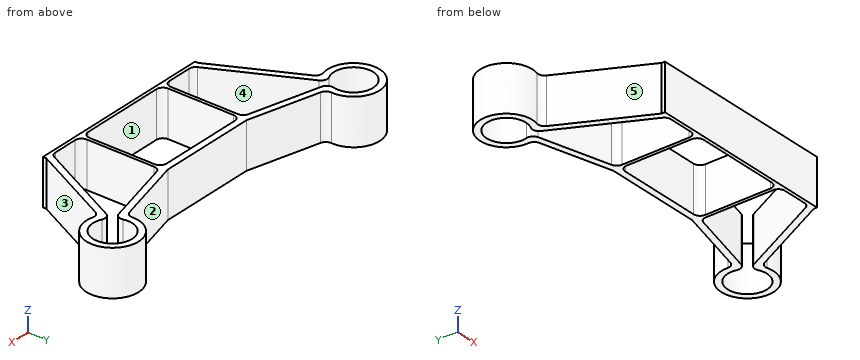
```python
from build123d import *

# Parameters (mm, degrees)
F1_DEPTH = 7
F2_R     = 1
F3_R     = 1


with BuildPart() as f1:
    # F0 (on Top) → F1 (new body)
    with BuildSketch(Plane.XY):
        with BuildLine():
            ThreePointArc((20.490715, 21.30806), (25.314352, 24.866528), (20.822566, 20.897394))
            Line((20.822566, 20.897394), (13.382216, 6))
            Line((13.382216, 6), (14.5, 6))
            Line((14.5, 6), (21.19372, 19.40246))
            ThreePointArc((21.19372, 19.40246), (26.092146, 25.495048), (19.107008, 21.984771))
            Line((19.107008, 21.984771), (7.5, 19))
            Line((7.5, 19), (0, 19))
            Line((0, 19), (0, 18))
            Line((0, 18), (7.5, 18))
            Line((7.5, 18), (7.626518, 18))
            Line((7.626518, 18), (8, 18.096042))
            Line((8, 18.096042), (20.490715, 21.30806))
        make_face()
        Polygon((14.5, 6), (13.382216, 6), (8, 6), (7.5, 6), (0, 6), (0, 5.5), (14.5, 5.5), align=None)
        Polygon((8, 6), (8, 18.096042), (7.626518, 18), (7.5, 18), (7.5, 6), align=None)
    extrude(amount=F1_DEPTH)

    # F2
    f2_edges = [f1.edges().sort_by_distance(p)[0] for p in [
        (21.19372, 19.40246, 3.5),
        (20.822566, 20.897394, 3.5),
        (20.490715, 21.30806, 3.5),
        (19.107008, 21.984771, 3.5),
    ]]
    fillet(f2_edges, radius=F2_R)

    # F3
    f3_edges = [f1.edges().sort_by_distance(p)[0] for p in [
        (8, 18.096042, 3.5),
        (13.382216, 6, 3.5),
        (8, 6, 3.5),
        (7.5, 18, 3.5),
        (7.5, 6, 3.5),
    ]]
    fillet(f3_edges, radius=F3_R)

    # F4: F1 across plane


with BuildPart() as f1_1:
    add(f1.part)
    add(f1.part.mirror(Plane.YZ))


solid = f1_1.part
```
Design review of the part built by this model. Coordinates are the model's own, in mm. Face numbers are marked on the shaded views. A direction names the side the tool comes from. Round coordinates to 2 decimals unless told otherwise and drop trailing zeros. Write each loop counter-clockwise with the first axis right and the second up, starting at its lowest first coordinate (ties: lowest second). Pieces come first, ordered by that corner, then holes. Notation, with made-up numbers: (-8.5, 40) -> (39.5, 40) arc R22 cw to (39.5, 59) -> close; hole circle Ø1 at (33, 85.5). An arc over 180 degrees is marked (long way). Answer in a Markdown table with one row per item.
Q1. To check wall thickness, follow L1, parallel to X at y = 11.5, z = 4.5; L2, parallel to Y at x = 3, z = 0.75; L3, parallel to X at y = 24.25, z = 6. State the ranges of each line that lie inside material, in increasing order. Write a range as [from, to].
The answers:
| item | result |
|---|---|
| L1 | [-17.25, -16.13], [-8, -7.5], [7.5, 8], [16.13, 17.25] |
| L2 | [5.5, 6], [18, 19] |
| L3 | [-26.77, -25.7], [-20.26, -19.19], [19.19, 20.26], [25.7, 26.77] |
Q2. Take a section at B-B, the plane y = 23.25. State the section outline as (x, z) points, then the cut area to 3 significant figures.
The answers:
| item | result |
|---|---|
| outline | (-26.97, 0) -> (-25.97, 0) -> (-25.97, 7) -> (-26.97, 7) -> close; (-19.99, 0) -> (-18.99, 0) -> (-18.99, 7) -> (-19.99, 7) -> close; (18.99, 0) -> (19.99, 0) -> (19.99, 7) -> (18.99, 7) -> close; (25.97, 0) -> (26.97, 0) -> (26.97, 7) -> (25.97, 7) -> close |
| area | 28.1 mm² |
Q3. Take a section at D-D, the plane y = 16.25. State the section outline as (x, z) points, then the cut area to 3 significant figures.
The answers:
| item | result |
|---|---|
| outline | (-19.62, 0) -> (-18.5, 0) -> (-18.5, 7) -> (-19.62, 7) -> close; (-8, 0) -> (-7.5, 0) -> (-7.5, 7) -> (-8, 7) -> close; (7.5, 0) -> (8, 0) -> (8, 7) -> (7.5, 7) -> close; (18.5, 0) -> (19.62, 0) -> (19.62, 7) -> (18.5, 7) -> close |
| area | 22.6 mm² |
Q4. Take a section at A-A, the plane x = 1. State the section outline as (y, z) points, then the cut area to 3 significant figures.
The answers:
| item | result |
|---|---|
| outline | (5.5, 0) -> (6, 0) -> (6, 7) -> (5.5, 7) -> close; (18, 0) -> (19, 0) -> (19, 7) -> (18, 7) -> close |
| area | 10.5 mm² |
Q5. For the marked faces 1 and 2, list the 3-axis set-ups (+Z, -Z, +X, -X, +Y, -Y) from which the entire face can be reached by the end or side of a thin tool; tool diameter is ignored.
The answers:
| item | result |
|---|---|
| face 1 | +Z, -Z |
| face 2 | +Z, -Z, +Y |
Q6. Clearance check with flat-ended pins moving along their axes: pin 1 Ø1.5 at (x, y) = (-15, 19) entering from +Z; pin 2 Ø3.5 at (y, z) = (13, 3.5) entering from -X; pin 3 Ø1.1 at (x, z) = (10.5, 4.5) entering from +Y; pin 4 Ø3 at (x, z) = (-11, 2.5) entering from +Y. State where each tip first meets the part, or that it passes through.
The answers:
| item | result |
|---|---|
| pin 1 | through |
| pin 2 | x = -18.87 |
| pin 3 | y = 19.91 |
| pin 4 | y = 20.29 |
Q7. Take a section at C-C, the plane x = 7. State the section outline as (y, z) points.
The answers:
| item | result |
|---|---|
| outline | (5.5, 0) -> (6.13, 0) -> (6.13, 7) -> (5.5, 7) -> close; (17.87, 0) -> (19, 0) -> (19, 7) -> (17.87, 7) -> close |
Q8. Draft analysis for pull direction X (two halves, no side actions). For the marked faces 3, 4 and 5, state which applies: +X half, -X half, draft (parallel to the pull), parting line (faces both ways), or undercut.
The answers:
| item | result |
|---|---|
| face 3 | +X half |
| face 4 | undercut |
| face 5 | -X half |
